Could you check a few things on this model? Use its own coordinates, in mm. A direction names the side the tool comes from. Round coordinates to 2 decimals unless told otherwise and drop trailing zeros. Loops run counter-clockwise (first coordinate to the right, second up) from the corner with the lowest first, then second, coordinate; pieces in that order, holes last. Notation, with made-up numbers: (1.5, 56.5) -> (19.5, 56.5) arc R31 cw to (19.5, 92.5) -> close; hole circle Ø4 at (18, 16). An arc over 180 degrees is marked (long way). One line per item, written item: value.
```python
from build123d import *

# Parameters (mm, degrees)
F0_R     = 44.45
F1_DEPTH = 19.05
F2_R     = 63.5
F2_R_2   = 44.45
F3_DEPTH = 107.95
F4_W     = 254
F4_H     = 50.8
F5_DEPTH = 127
F6_W     = 25.4
F6_H     = 99.06
F7_DEPTH = 88.9


with BuildPart() as f1:
    # F0 (on Front) → F1 (new body)
    with BuildSketch(Plane.XZ):
        with BuildLine():
            Line((127, -152.4), (59.227747, 22.898122))
            ThreePointArc((59.227747, 22.898122), (0, 63.5), (-59.227747, 22.898122))
            Line((-59.227747, 22.898122), (-127, -152.4))
            Line((-127, -152.4), (-127, -203.2))
            Line((-127, -203.2), (127, -203.2))
            Line((127, -203.2), (127, -152.4))
        make_face()
        Circle(F0_R, mode=Mode.SUBTRACT)
    extrude(amount=F1_DEPTH)

    # F2 (on face) → F3 (join)
    with BuildSketch(Plane.XZ.offset(19.05)):
        Circle(F2_R)
        Circle(F2_R_2, mode=Mode.SUBTRACT)
    extrude(amount=F3_DEPTH)

    # F4 (on face) → F5 (join)
    with BuildSketch(Plane.XZ.offset(19.05)):
        with Locations((0, -177.8)):
            Rectangle(F4_W, F4_H)
    extrude(amount=F5_DEPTH)

    # F6 (on face) → F7 (join)
    with BuildSketch(Plane.XZ.offset(19.05)):
        with Locations((0, -102.87)):
            Rectangle(F6_W, F6_H)
    extrude(amount=F7_DEPTH)


solid = f1.part
```
(1) We'd pull the mould along Z, two halves only. Please class faces 1 (the face through (93.59, -9.39, -65.98)), 2 (the face through (-43, -127, -13)), 3 (the face through (42.397, -62.611, 13.352)): +Z half, -Z half, draft (parallel to the pull), parting line (faces both ways), or undercut.
Results below:
face 1: +Z half
face 2: draft
face 3: undercut
(2) For pin 1 Ø1 at (y, z) = (-76, -46.5) entering from -X (3 decimals); pin 2 Ø10 at (x, y) = (19, -88) entering from +Z; pin 3 Ø20.5 at (x, z) = (6, -97.5) entering from -Y, each with a flat end and sliding along its axis, tell me the tip position at first contact or that it passes through.
Results below:
pin 1: stops at x = -43.775
pin 2: stops at z = 61.94
pin 3: stops at y = -107.95
(3) Please list where these lines run through material, in increasing order: L1, parallel to Z at x = -24.5, y = -57; L2, parallel to Z at x = 0, y = -46; L3, parallel to Y at x = 35.5, z = -76.
Results below:
L1: z = -203.2 to -152.4, -58.58 to -37.09, 37.09 to 58.58
L2: z = -203.2 to -44.45, 44.45 to 63.5
L3: y = -19.05 to 0
(4) Imagine slicing it at A-A on y = -98. Write out the boundary of the cut face in (x, z), then the cut area to 3 significant figures.
Results below:
outline: (-127, -203.2) -> (127, -203.2) -> (127, -152.4) -> (12.7, -152.4) -> (12.7, -62.22) arc R63.5 ccw (long way) to (-12.7, -62.22) -> (-12.7, -152.4) -> (-127, -152.4) -> close; hole circle Ø88.9 at (0, 0)
area: 21,600 mm²
(5) Imagine slicing it at C-C on z = 0. Write out the boundary of the cut face in (x, y), then the cut area to 3 significant figures.
Results below:
outline: (-68.08, -19.05) -> (-63.5, -19.05) -> (-63.5, -127) -> (-44.45, -127) -> (-44.45, 0) -> (-68.08, 0) -> close; (44.45, -127) -> (63.5, -127) -> (63.5, -19.05) -> (68.08, -19.05) -> (68.08, 0) -> (44.45, 0) -> close
area: 5,010 mm²
(6) On a 3-axis mill with a long thin cutter (end or side, diameter ignored), from which of +Z, -Z, +X, -X, +Y, -Y can I reach the whole of each face in a straight line? I mean faces 4 (the face through (-127, -72, -178)), 5 (the face through (-2, -110, -152.4)), 6 (the face through (12.7, -63, -108)), 7 (the face through (-58, -19.05, -102)). Say none if no direction works.
Results below:
face 4: +Z, -Z, -X, +Y, -Y
face 5: -Y
face 6: +X, -Y
face 7: -X, -Y
(7) Imagine slicing it at B-B on x = 0. Write out the boundary of the cut face in (y, z).
Results below:
outline: (-146.05, -203.2) -> (0, -203.2) -> (0, -44.45) -> (-127, -44.45) -> (-127, -63.5) -> (-107.95, -63.5) -> (-107.95, -152.4) -> (-146.05, -152.4) -> close; (-127, 44.45) -> (0, 44.45) -> (0, 63.5) -> (-127, 63.5) -> close
(8) Imagine slicing it at D-D on z = -48.5. Write out the boundary of the cut face in (x, y), then the cut area to 3 significant figures.
Results below:
outline: (-86.83, -19.05) -> (-40.99, -19.05) -> (-40.99, -127) -> (40.99, -127) -> (40.99, -19.05) -> (86.83, -19.05) -> (86.83, 0) -> (-86.83, 0) -> close
area: 12,200 mm²
